from build123d import *

# Parameters (mm, degrees)
F1_DEPTH = 880
F2_T     = -16


with BuildPart() as f1:
    # F0 (on Top) → F1 (new body)
    with BuildSketch(Plane.XY):
        Polygon((-570, 0), (0, 0), (0, -380), (350, -380), (350, 560), (-570, 560), align=None)
    extrude(amount=F1_DEPTH)

    # F2
    f2_openings = [f1.faces().sort_by_distance(p)[0] for p in [
        (-110, 560, 440),
        (350, 90, 440),
        (-51.522678, 183.563715, 0),
    ]]
    offset(amount=F2_T, openings=f2_openings, kind=Kind.INTERSECTION)


solid = f1.part
Input: part model. Units: mm. Frame: model coordinates. A direction names the side the tool comes from. Coordinates: 2 decimals unless noted, no trailing zeros. Loops run counter-clockwise (first coordinate to the right, second up) from the corner with the lowest first, then second, coordinate; pieces in that order, holes last. Notation, with made-up numbers: (-3.75, -20.75) - (30.25, -20.75) arc R26 cw to (30.25, -2.75) - close; hole circle Ø9 at (1.5, 15.5). An arc over 180 degrees is marked (long way). Answer in a Markdown table with one row per item. Add a question column.
Item 1: Line query: line 1 along Z through (x, y) = (201.5, -107); line 2 along Y through (x, z) = (-432.5, 312). Output: solid intervals per line, ascending. Write a range as [from, to].
Item 2: Contact query for flat-ended pins moving along their axis: P1, Ø12, axis at x = -175.5, z = 228, coming from the -Y side; P2, Ø8, axis at y = -21.5, z = 335.5, coming from the -X side; P3, Ø6, axis at x = 72, z = 278, coming from the +Y side. Output: stop coordinate, or through.
Item 3: Section query A-A on y = -132. Return the cut outline in (x, z), then the cut area to 3 significant figures.
Item 4: Section query C-C on z = 676.5. Return the cut outline in (x, y), then the cut area to 3 significant figures.
Item 5: Access query for faces 1 (the flat face through (16, -171, 426)), 2 (the flat face through (-14, 201, 880)), 3 (the flat face through (0, -187, 434)). Directions: +Z, -Z, +X, -X, +Y, -Y. A direction counts if a zero-diameter tool reaches every point of the face in a straight line with its end or side. Return the directions, or none.
Item 6: Section query B-B on x = 241.5. Return the cut outline in (y, z), then the cut area to 3 significant figures.
Recorded:
| question | item | result |
|---|---|---|
| 1 | line 1 | [864, 880] |
| 1 | line 2 | [0, 16] |
| 2 | P1 | y = 0 |
| 2 | P2 | x = 0 |
| 2 | P3 | y = -364 |
| 3 | outline | (0, 0) - (16, 0) - (16, 864) - (350, 864) - (350, 880) - (0, 880) - close |
| 3 | area | 19,400 mm^2 |
| 4 | outline | (-570, 0) - (0, 0) - (0, -380) - (350, -380) - (350, -364) - (16, -364) - (16, 16) - (-554, 16) - (-554, 560) - (-570, 560) - close |
| 4 | area | 29,500 mm^2 |
| 5 | face 1 | -Z, +X, +Y |
| 5 | face 2 | +Z, +X, -X, +Y, -Y |
| 5 | face 3 | +Z, -Z, -X, -Y |
| 6 | outline | (-380, 0) - (-364, 0) - (-364, 864) - (560, 864) - (560, 880) - (-380, 880) - close |
| 6 | area | 28,900 mm^2 |
